Design review of the part built by this model. Coordinates are the model's own, in mm. Give positions to 0.01 mm unless a question says otherwise; leave off trailing zeros. Loops run counter-clockwise (first coordinate to the right, second up) from the corner with the lowest first, then second, coordinate; pieces in that order, holes last. Notation, with made-up numbers: (67.5, 32) - (92.5, 32) arc R10 cw to (92.5, 48) - close; hole circle Ø8 at (-10.5, 49). An arc over 180 degrees is marked (long way). Write each question's results on one line, items separated by ' | '.
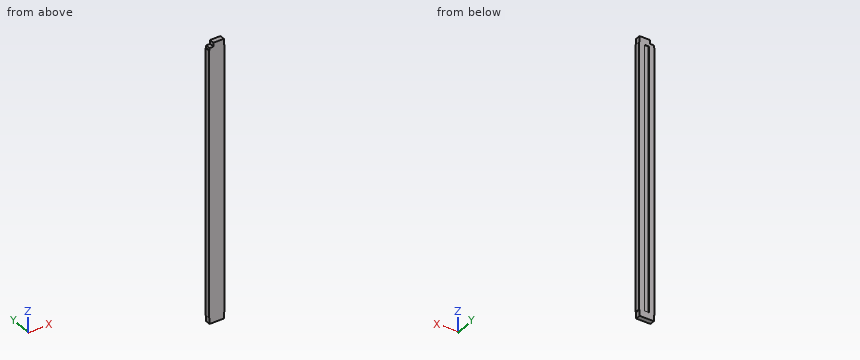
```python
from build123d import *

# Parameters (mm, degrees)
SKETCH1_W               = 12.7
SKETCH1_H               = 4.064
BOSS_EXTRUDE1_DEPTH     = 228.6
SKETCH2_W               = 3.429
SKETCH2_H               = 217.3732
CUT_EXTRUDE1_DEPTH      = 0.254
SKETCH3_W               = 0.508
SKETCH3_H               = 5.08
CUT_EXTRUDE2_DEPTH      = 229.724285103
MIRROR2_COPY_1_SKETCH_W = 0.508
MIRROR2_COPY_1_SKETCH_H = 5.08
MIRROR2_COPY_1_DEPTH    = 229.724285103
SKETCH4_W               = 3.175
SKETCH4_H               = 3.175
CUT_EXTRUDE3_DEPTH      = 229.724285103


with BuildPart() as part:
    # Sketch1 → Boss-Extrude1 (new body)
    with BuildSketch(Plane.XY):
        Rectangle(SKETCH1_W, SKETCH1_H)
    extrude(amount=BOSS_EXTRUDE1_DEPTH)

    # Sketch2 → Cut-Extrude1 (cut)
    with BuildSketch(Plane(origin=(0, 2.032, 0), x_dir=(1, 0, 0), z_dir=(0, 1, 0))):
        with Locations((0, -114.3)):
            Rectangle(SKETCH2_W, SKETCH2_H)
    extrude(amount=-CUT_EXTRUDE1_DEPTH, mode=Mode.SUBTRACT)

    # Sketch3 → Cut-Extrude2 (cut, through all)
    with BuildSketch(Plane(origin=(0, 2.032, 0), x_dir=(1, 0, 0), z_dir=(0, 1, 0))):
        with Locations((-6.096, -226.06)):
            Rectangle(SKETCH3_W, SKETCH3_H)
    cut_extrude2 = extrude(amount=-CUT_EXTRUDE2_DEPTH, mode=Mode.SUBTRACT)

    # Mirror1: Cut-Extrude2 across plane
    add(cut_extrude2.mirror(Plane(origin=(0, 0, 114.3), x_dir=(1, 0, 0), z_dir=(0, 0, -1))), mode=Mode.SUBTRACT)

    # Mirror2: Cut-Extrude2 across plane
    add(cut_extrude2.mirror(Plane(origin=(0, 0, 0), x_dir=(0, 0, 1), z_dir=(1, 0, 0))), mode=Mode.SUBTRACT)

    # Mirror2 copy 1 sketch → Mirror2 copy 1 (cut, through all)
    with BuildSketch(Plane(origin=(0, 2.032, 228.6), x_dir=(-1, 0, 0), z_dir=(0, 1, 0))):
        with Locations((-6.096, -226.06)):
            Rectangle(MIRROR2_COPY_1_SKETCH_W, MIRROR2_COPY_1_SKETCH_H)
    extrude(amount=-MIRROR2_COPY_1_DEPTH, mode=Mode.SUBTRACT)

    # Sketch4 → Cut-Extrude3 (cut, through all)
    with BuildSketch(Plane(origin=(0, 2.032, 0), x_dir=(1, 0, 0), z_dir=(0, 1, 0))):
        with Locations((-4.2545, -227.0125)):
            Rectangle(SKETCH4_W, SKETCH4_H)
    extrude(amount=-CUT_EXTRUDE3_DEPTH, mode=Mode.SUBTRACT)


solid = part.part
```
Item 1: We need section A-A on z = 37. Give the boundary of the cut face in (x, y).
Output values:
outline: (-6.35, -2.03) - (6.35, -2.03) - (6.35, 2.03) - (1.71, 2.03) - (1.71, 1.78) - (-1.71, 1.78) - (-1.71, 2.03) - (-6.35, 2.03) - close
Item 2: Clearance check with flat-ended pins moving along their axes: P1, Ø2, axis at y = 0, z = 226, coming from the +X side; P2, Ø0.6, axis at y = -1, z = 225, coming from the -X side. State where each tip first meets the part, or that it passes through.
Output values:
P1: stops at x = 5.84 | P2: stops at x = -5.84
Item 3: Wall thickness on probe 1 along X at (y, z) = (1.85, 59.5); probe 2 along Y at (x, z) = (1.5, 179.5); probe 3 along Z at (x, y) = (-5.75, 1.2) (3 decimals): over which ranges is each line inside the solid? List them lowest first.
Output values:
probe 1: x = -6.35 to -1.71, 1.71 to 6.35 | probe 2: y = -2.03 to 1.78 | probe 3: z = 0 to 225.425
